```python
from build123d import *

# Parameters (mm, degrees)
F0_W     = 34
F0_H     = 17.8
F1_DEPTH = 5
F3_D     = 2
F5_D     = 2
F7_D     = 3


with BuildPart() as f1:
    # F0 (on Top) → F1 (new body)
    with BuildSketch(Plane.XY):
        Rectangle(F0_W, F0_H)
    extrude(amount=-F1_DEPTH)

    # F3 (through all)
    with Locations(Plane.XY):
        with Locations((-13, 0)):
            Hole(F3_D / 2)

    # F5 (through all)
    with Locations(Plane.XY):
        with Locations((13, 0)):
            Hole(F5_D / 2)

    # F7 (through all)
    with Locations(Plane.XY):
        with Locations((-9.5, -4.9), (-5.5, -4.9), (-1.5, -4.9), (2.5, -4.9), (6.5, -4.9), (10.5, -4.9)):
            Hole(F7_D / 2)


solid = f1.part
```
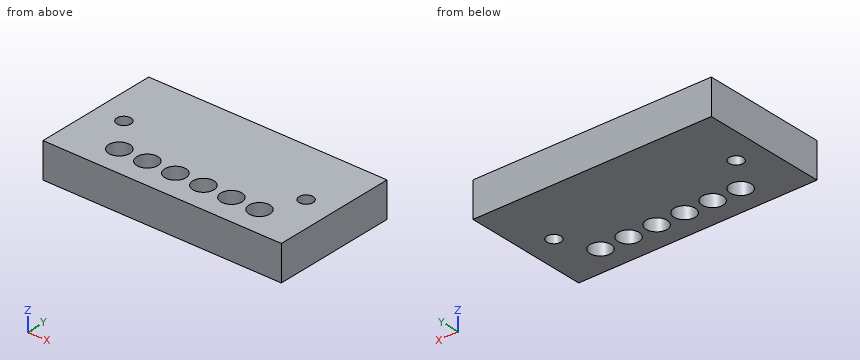
CAD build for the part. Positions are in the model's coordinates, mm. Coordinates: 2 decimals unless noted, no trailing zeros. Order: outer loops, then holes, each group sorted by start corner. A loop starts at its lowest first (then second) coordinate and runs counter-clockwise, first axis right, second up. Notation, with made-up numbers: (3.25, -19.75) - (58.25, -19.75) arc R18 ccw to (58.25, -4.75) - close; hole circle Ø11 at (-16, 29). An arc over 180 degrees is marked (long way). Answer in a Markdown table with one row per item.
1. Slice it at D-D, the plane x = -13. List the corners of the cut face in (y, z).
Answer:
| item | result |
|---|---|
| outline | (-8.9, -5) - (-1, -5) - (-1, 0) - (-8.9, 0) - close; (1, -5) - (8.9, -5) - (8.9, 0) - (1, 0) - close |
2. Flat gauge pin, fed straight in: P1, Ø2.5, axis at x = 10.5, y = -4.9, coming from the -Z side. Where does the tip first touch, or does it go through?
Answer:
| item | result |
|---|---|
| P1 | through |
3. Slice it at A-A, the plane y = 0. List the corners of the cut face in (x, z).
Answer:
| item | result |
|---|---|
| outline | (-17, -5) - (-14, -5) - (-14, 0) - (-17, 0) - close; (-12, -5) - (12, -5) - (12, 0) - (-12, 0) - close; (14, -5) - (17, -5) - (17, 0) - (14, 0) - close |
4. Drill centre lines: L1, parallel to Y at x = -1.5, z = -2.7; L2, parallel to Y at x = -13, z = -2.75; L3, parallel to X at y = -0.5, z = -4.7. Where is each one in solid material? Low to high. Write a range as from..to.
Answer:
| item | result |
|---|---|
| L1 | -8.9..-6.4, -3.4..8.9 |
| L2 | -8.9..-1, 1..8.9 |
| L3 | -17..-13.87, -12.13..12.13, 13.87..17 |
5. Slice it at C-C, the plane z = -1.2. Give the number of separate pieces and of enclosed holes in the cut face, then the cut area to 3 significant figures.
Answer:
| item | result |
|---|---|
| separate pieces | 1 |
| enclosed holes | 8 |
| area | 557 mm² |
6. Slice it at B-B, the plane x = 6.5. List the corners of the cut face in (y, z), then the cut area to 3 significant figures.
Answer:
| item | result |
|---|---|
| outline | (-8.9, -5) - (-6.4, -5) - (-6.4, 0) - (-8.9, 0) - close; (-3.4, -5) - (8.9, -5) - (8.9, 0) - (-3.4, 0) - close |
| area | 74.0 mm² |
